The model under review builds one solid part; all positions refer to its coordinate system, in mm. A direction names the side the tool comes from. Give positions to 0.01 mm unless a question says otherwise; leave off trailing zeros. Order: outer loops, then holes, each group sorted by start corner. A loop starts at its lowest first (then second) coordinate and runs counter-clockwise, first axis right, second up.
```python
from build123d import *

# Parameters (mm, degrees)
EXTRUDE_1_DEPTH = 60


with BuildPart() as part:
    # Model → 凸台-拉伸1 (new body)
    with BuildSketch(Plane.XY):
        with BuildLine():
            ThreePointArc((-26.623667603, 4.492251481), (-24.628342026, 3.167806143), (-22.375329871, 2.355761908))
            ThreePointArc((-22.375329871, 2.355761908), (-22.454603363, 1.412723899), (-22.494148969, 0.467186424))
            ThreePointArc((-22.494148969, 0.467186424), (-24.83117158, -0.056077302), (-26.976760436, -1.119998387))
            ThreePointArc((-26.976760436, -1.119998387), (-26.946721668, -1.695344027), (-26.904413642, -2.269917752))
            ThreePointArc((-26.904413642, -2.269917752), (-24.642398725, -3.056535912), (-22.258221901, -3.282766946))
            ThreePointArc((-22.258221901, -3.282766946), (-22.100480854, -4.215892197), (-21.903638454, -5.141558466))
            ThreePointArc((-21.903638454, -5.141558466), (-24.037108806, -6.229576789), (-25.850703628, -7.793659087))
            ThreePointArc((-25.850703628, -7.793659087), (-25.67852594, -8.343458848), (-25.494656424, -8.889459704))
            ThreePointArc((-25.494656424, -8.889459704), (-23.108082884, -9.088824574), (-20.742547988, -8.715027478))
            ThreePointArc((-20.742547988, -8.715027478), (-20.357703853, -9.579608281), (-19.93684178, -10.427240328))
            ThreePointArc((-19.93684178, -10.427240328), (-21.732706083, -12.011649055), (-23.100352038, -13.977615523))
            ThreePointArc((-23.100352038, -13.977615523), (-22.796853989, -14.467323464), (-22.48297618, -14.95044421))
            ThreePointArc((-22.48297618, -14.95044421), (-20.12180121, -14.550028962), (-17.9235435, -13.599690783))
            ThreePointArc((-17.9235435, -13.599690783), (-17.335777449, -14.341402345), (-16.717340013, -15.057740331))
            ThreePointArc((-16.717340013, -15.057740331), (-18.06275751, -17.038985236), (-18.898520373, -19.28330697))
            ThreePointArc((-18.898520373, -19.28330697), (-18.48277186, -19.68215294), (-18.058607856, -20.072037323))
            ThreePointArc((-18.058607856, -20.072037323), (-15.871192762, -19.097001519), (-13.978336856, -17.6298355))
            ThreePointArc((-13.978336856, -17.6298355), (-13.224580391, -18.202073356), (-12.447426292, -18.742107131))
            ThreePointArc((-12.447426292, -18.742107131), (-13.257859452, -20.995699309), (-13.509225169, -23.377357322))
            ThreePointArc((-13.509225169, -23.377357322), (-13.007349201, -23.660280361), (-12.499550786, -23.932430511))
            ThreePointArc((-12.499550786, -23.932430511), (-10.623338904, -22.444039237), (-9.154819898, -20.552232814))
            ThreePointArc((-9.154819898, -20.552232814), (-8.282434311, -20.919041156), (-7.395394998, -21.248838411))
            ThreePointArc((-7.395394998, -21.248838411), (-7.619921326, -23.633176378), (-7.271095664, -26.002522336))
            ThreePointArc((-7.271095664, -26.002522336), (-6.714626953, -26.15174535), (-6.15510097, -26.289061072))
            ThreePointArc((-6.15510097, -26.289061072), (-4.707981592, -24.380835426), (-3.756071937, -22.183257755))
            ThreePointArc((-3.756071937, -22.183257755), (-2.819872422, -22.321588665), (-1.878683838, -22.420427026))
            ThreePointArc((-1.878683838, -22.420427026), (-1.503195518, -24.785694058), (-0.576096477, -26.993853242))
            ThreePointArc((-0.576096477, -26.993853242), (0, -27), (0.576096477, -26.993853242))
            ThreePointArc((0.576096477, -26.993853242), (1.503195518, -24.785694058), (1.878683838, -22.420427026))
            ThreePointArc((1.878683838, -22.420427026), (2.819872422, -22.321588665), (3.756071937, -22.183257755))
            ThreePointArc((3.756071937, -22.183257755), (4.707981592, -24.380835426), (6.15510097, -26.289061072))
            ThreePointArc((6.15510097, -26.289061072), (6.714626953, -26.15174535), (7.271095664, -26.002522336))
            ThreePointArc((7.271095664, -26.002522336), (7.619921325, -23.633176378), (7.395394998, -21.248838411))
            ThreePointArc((7.395394998, -21.248838411), (8.282434311, -20.919041156), (9.154819898, -20.552232814))
            ThreePointArc((9.154819898, -20.552232814), (10.623338904, -22.444039237), (12.499550786, -23.932430511))
            ThreePointArc((12.499550786, -23.932430511), (13.007349201, -23.660280361), (13.509225169, -23.377357322))
            ThreePointArc((13.509225169, -23.377357322), (13.257859452, -20.995699309), (12.447426292, -18.742107131))
            ThreePointArc((12.447426292, -18.742107131), (13.224580391, -18.202073356), (13.978336856, -17.6298355))
            ThreePointArc((13.978336856, -17.6298355), (15.871192762, -19.097001519), (18.058607856, -20.072037323))
            ThreePointArc((18.058607856, -20.072037323), (18.48277186, -19.68215294), (18.898520373, -19.28330697))
            ThreePointArc((18.898520373, -19.28330697), (18.06275751, -17.038985236), (16.717340013, -15.057740331))
            ThreePointArc((16.717340013, -15.057740331), (17.335777449, -14.341402345), (17.9235435, -13.599690783))
            ThreePointArc((17.9235435, -13.599690783), (20.12180121, -14.550028962), (22.48297618, -14.95044421))
            ThreePointArc((22.48297618, -14.95044421), (22.796853989, -14.467323464), (23.100352038, -13.977615523))
            ThreePointArc((23.100352038, -13.977615523), (21.732706083, -12.011649055), (19.93684178, -10.427240328))
            ThreePointArc((19.93684178, -10.427240328), (20.357703853, -9.579608281), (20.742547988, -8.715027478))
            ThreePointArc((20.742547988, -8.715027478), (23.108082884, -9.088824574), (25.494656424, -8.889459704))
            ThreePointArc((25.494656424, -8.889459704), (25.67852594, -8.343458848), (25.850703628, -7.793659087))
            ThreePointArc((25.850703628, -7.793659087), (24.037108806, -6.229576789), (21.903638454, -5.141558466))
            ThreePointArc((21.903638454, -5.141558466), (22.100480854, -4.215892197), (22.258221901, -3.282766946))
            ThreePointArc((22.258221901, -3.282766946), (24.642398725, -3.056535912), (26.904413642, -2.269917752))
            ThreePointArc((26.904413642, -2.269917752), (26.946721668, -1.695344027), (26.976760436, -1.119998387))
            ThreePointArc((26.976760436, -1.119998387), (24.83117158, -0.056077302), (22.494148969, 0.467186424))
            ThreePointArc((22.494148969, 0.467186424), (22.454603363, 1.412723899), (22.375329871, 2.355761907))
            ThreePointArc((22.375329871, 2.355761907), (24.628342026, 3.167806143), (26.623667603, 4.492251481))
            ThreePointArc((26.623667603, 4.492251481), (26.52175577, 5.059295494), (26.407768172, 5.624035931))
            ThreePointArc((26.407768172, 5.624035931), (24.065000522, 6.120945728), (21.671269376, 6.046576272))
            ThreePointArc((21.671269376, 6.046576272), (21.39782056, 6.952573356), (21.086513575, 7.846269576))
            ThreePointArc((21.086513575, 7.846269576), (23.066796021, 9.193103287), (24.670058614, 10.972156033))
            ThreePointArc((24.670058614, 10.972156033), (24.430330417, 11.496040872), (24.179478714, 12.014691387))
            ThreePointArc((24.179478714, 12.014691387), (21.786736975, 11.913367227), (19.486704228, 11.246037495))
            ThreePointArc((19.486704228, 11.246037495), (18.996533996, 12.05556706), (18.47275408, 12.843767271))
            ThreePointArc((18.47275408, 12.843767271), (20.055878388, 14.640763942), (21.166339111, 16.762639667))
            ThreePointArc((21.166339111, 16.762639667), (20.803857555, 17.210447723), (20.431903681, 17.650419597))
            ThreePointArc((20.431903681, 17.650419597), (18.139532619, 16.957228049), (16.077717785, 15.738868823))
            ThreePointArc((16.077717785, 15.738868823), (15.401625336, 16.401065148), (14.698283508, 17.034243832))
            ThreePointArc((14.698283508, 17.034243832), (15.784776155, 19.168491554), (16.332660679, 21.499865003))
            ThreePointArc((16.332660679, 21.499865003), (15.870201812, 21.843458848), (15.400516998, 22.17710703))
            ThreePointArc((15.400516998, 22.17710703), (13.352554715, 20.935603868), (11.658509204, 19.242769139))
            ThreePointArc((11.658509204, 19.242769139), (10.838975914, 19.716023994), (10.000265727, 20.154396205))
            ThreePointArc((10.000265727, 20.154396205), (10.521858385, 22.491792344), (10.472741108, 24.88617475))
            ThreePointArc((10.472741108, 24.88617475), (9.939362922, 25.103965119), (9.401459192, 25.310325266))
            ThreePointArc((9.401459192, 25.310325266), (7.726586692, 23.5985187), (6.506753613, 21.5375755))
            ThreePointArc((6.506753613, 21.5375755), (5.595273771, 21.792152542), (4.673894472, 22.008173742))
            ThreePointArc((4.673894472, 22.008173742), (4.597813555, 24.401851103), (3.954780698, 26.708794612))
            ThreePointArc((3.954780698, 26.708794612), (3.383997306, 26.787096935), (2.811673129, 26.853202681))
            ThreePointArc((2.811673129, 26.853202681), (1.61512881, 24.778651813), (0.946154762, 22.479096783))
            ThreePointArc((0.946154762, 22.479096783), (0, 22.499), (-0.946154762, 22.479096783))
            ThreePointArc((-0.946154762, 22.479096783), (-1.61512881, 24.778651813), (-2.811673129, 26.853202681))
            ThreePointArc((-2.811673129, 26.853202681), (-3.383997306, 26.787096935), (-3.954780698, 26.708794612))
            ThreePointArc((-3.954780698, 26.708794612), (-4.597813555, 24.401851103), (-4.673894472, 22.008173742))
            ThreePointArc((-4.673894472, 22.008173742), (-5.595273771, 21.792152542), (-6.506753613, 21.5375755))
            ThreePointArc((-6.506753613, 21.5375755), (-7.726586692, 23.5985187), (-9.401459192, 25.310325266))
            ThreePointArc((-9.401459192, 25.310325266), (-9.939362922, 25.103965119), (-10.472741108, 24.88617475))
            ThreePointArc((-10.472741108, 24.88617475), (-10.521858385, 22.491792344), (-10.000265727, 20.154396205))
            ThreePointArc((-10.000265727, 20.154396205), (-10.838975914, 19.716023994), (-11.658509204, 19.242769139))
            ThreePointArc((-11.658509204, 19.242769139), (-13.352554715, 20.935603868), (-15.400516998, 22.17710703))
            ThreePointArc((-15.400516998, 22.17710703), (-15.870201812, 21.843458848), (-16.332660679, 21.499865003))
            ThreePointArc((-16.332660679, 21.499865003), (-15.784776155, 19.168491554), (-14.698283508, 17.034243832))
            ThreePointArc((-14.698283508, 17.034243832), (-15.401625336, 16.401065148), (-16.077717785, 15.738868823))
            ThreePointArc((-16.077717785, 15.738868823), (-18.139532619, 16.957228049), (-20.431903682, 17.650419597))
            ThreePointArc((-20.431903682, 17.650419597), (-20.803857555, 17.210447723), (-21.166339111, 16.762639667))
            ThreePointArc((-21.166339111, 16.762639667), (-20.055878388, 14.640763942), (-18.47275408, 12.843767271))
            ThreePointArc((-18.47275408, 12.843767271), (-18.996533996, 12.05556706), (-19.486704227, 11.246037495))
            ThreePointArc((-19.486704227, 11.246037495), (-21.786736975, 11.913367227), (-24.179478714, 12.014691387))
            ThreePointArc((-24.179478714, 12.014691387), (-24.430330417, 11.496040872), (-24.670058614, 10.972156033))
            ThreePointArc((-24.670058614, 10.972156033), (-23.066796021, 9.193103287), (-21.086513575, 7.846269576))
            ThreePointArc((-21.086513575, 7.846269576), (-21.39782056, 6.952573356), (-21.671269376, 6.046576272))
            ThreePointArc((-21.671269376, 6.046576272), (-24.065000522, 6.120945728), (-26.407768172, 5.624035931))
            ThreePointArc((-26.407768172, 5.624035931), (-26.52175577, 5.059295494), (-26.623667603, 4.492251481))
        make_face()
        with BuildLine():
            Line((5, 14.142135624), (5, 18.3))
            Line((5, 18.3), (-5, 18.3))
            Line((-5, 18.3), (-5, 14.142135624))
            ThreePointArc((-5, 14.142135624), (0, -15), (5, 14.142135624))
        make_face(mode=Mode.SUBTRACT)
    extrude(amount=EXTRUDE_1_DEPTH)


solid = part.part
```
1. Insertion check: pin 1 (1.5 mm diameter, centred on y = 4.5, z = 19, fed in from +X); pin 2 (12 mm diameter, centred on x = 12.5, z = 32, fed in from -Y); pin 3 (4 mm diameter, centred on y = -14.5, z = 26, fed in from -X). Each pin has a flat end and moves straight along its axis. Give the tip position at first contact, or say it passes through.
2. For faces 1 (the cylindrical face through (24.598, 3.153, 29.58)), 2 (the cylindrical face through (-15.9, -19.114, 29.58)), 3 (the cylindrical face through (-13.326, 20.915, 29.58)), 4 (the cylindrical face through (13.265, -21.028, 29.58)), list the 3-axis set-ups (+Z, -Z, +X, -X, +Y, -Y) from which the entire face can be reached by the end or side of a thin tool; tool diameter is ignored.
3. To check wall thickness, follow line 1 (Y direction, x = 0, z = 32); line 2 (Y direction, x = -24, z = 47); line 3 (X direction, y = 24, z = 51). State the ranges of each line that lie inside material, in increasing order.
4. Take a section at A-A (y = -16). Write out the cut boundary in (x, z), and give its area (3 significant figures).
Answer:
1. pin 1: stops at x = 26.62
1. pin 2: stops at y = -26.21
1. pin 3: stops at x = -23.1
2. face 1: +Z, -Z, +X
2. face 2: +Z, -Z, -Y
2. face 3: +Z, -Z, +Y
2. face 4: +Z, -Z
3. line 1: y = -27 to -15, 18.3 to 22.5
3. line 2: y = -9.08 to -6.2, -3.17 to 0.2, 2.88 to 6.13, 10.12 to 12.03
3. line 3: x = -10.56 to -8.05, -4.65 to -1.32, 1.32 to 4.65, 8.05 to 10.56
4. outline: (-17.44, 0) - (17.44, 0) - (17.44, 60) - (-17.44, 60) - close
4. area: 2,090 mm2
